Verification items for the finished model (mm, model axes). A direction names the side the tool comes from. Coordinates: 2 decimals unless noted, no trailing zeros. Loops run counter-clockwise (first coordinate to the right, second up) from the corner with the lowest first, then second, coordinate; pieces in that order, holes last. Notation, with made-up numbers: (-15, 16) -> (31, 16) arc R24 cw to (31, 26) -> close; hole circle Ø6 at (75, 9). An arc over 180 degrees is marked (long way). Write item = value, one per line.
```python
from build123d import *

# Parameters (mm, degrees)
CUT_EXTRUDE1_REACH   = 17
CUT_EXTRUDE2_REACH   = 17
CUT_EXTRUDE3_REACH   = 17
CUT_EXTRUDE4_REACH   = 16.83
M8_CLEARANCE_HOLE1_D = 8.917
CHAMFER1_SIZE        = 0.5415
FILLET1_R            = 0.3
FILLET2_R            = 1


with BuildPart() as part:
    # Sketch1 → Revolve1 (revolve)
    with BuildSketch(Plane(origin=(0, 0, 0), x_dir=(-1, 0, 0), z_dir=(0, 0, -1)), mode=Mode.PRIVATE) as revolve1_sk:
        Polygon((-5, 8), (-5, 0), (0, 0), (0, 10), (-3.701184814, 10), align=None)
    revolve(revolve1_sk.sketch.rotate(Axis((5, 0, 0), (-1, 0, 0)), 270), axis=Axis((5, 0, 0), (-1, 0, 0)))

    # Cut-Extrude1: up to this cone (the profile starts inside it)
    cut_extrude1_end = Plane(origin=(0, 0, 0), z_dir=(-1, 0, 0)).offset(-10.195259746) * Cone(1.54e-06, 66.821801925, 43.394584565, align=(Align.CENTER, Align.CENTER, Align.MIN), mode=Mode.PRIVATE)
    # Sketch2 → Cut-Extrude1 (cut, up to the surface)
    with BuildSketch(Plane.ZY, mode=Mode.PRIVATE) as cut_extrude1_sk1:
        with BuildLine():
            Line((9.743587635, 2.25), (8.2, 2.25))
            Line((8.2, 2.25), (8.2, -2.25))
            Line((8.2, -2.25), (9.743587635, -2.25))
            ThreePointArc((9.743587635, -2.25), (10, 0), (9.743587635, 2.25))
        make_face()
    cut_extrude1_tool1 = extrude(cut_extrude1_sk1.sketch, amount=-CUT_EXTRUDE1_REACH, mode=Mode.PRIVATE) & cut_extrude1_end
    add(cut_extrude1_tool1.solids().sort_by_distance((0, 0, 9.059184))[0], mode=Mode.SUBTRACT)

    # Cut-Extrude2: up to this cone (the profile starts inside it)
    cut_extrude2_end = Plane(origin=(0, 0, 0), z_dir=(-1, 0, 0)).offset(-10.195259746) * Cone(1.54e-06, 66.821801925, 43.394584565, align=(Align.CENTER, Align.CENTER, Align.MIN), mode=Mode.PRIVATE)
    # Sketch3 → Cut-Extrude2 (cut, up to the surface)
    with BuildSketch(Plane.ZY, mode=Mode.PRIVATE) as cut_extrude2_sk1:
        with BuildLine():
            Line((2.25, -9.743587635), (2.25, -8.2))
            Line((2.25, -8.2), (-2.25, -8.2))
            Line((-2.25, -8.2), (-2.25, -9.743587635))
            ThreePointArc((-2.25, -9.743587635), (0, -10), (2.25, -9.743587635))
        make_face()
    cut_extrude2_tool1 = extrude(cut_extrude2_sk1.sketch, amount=-CUT_EXTRUDE2_REACH, mode=Mode.PRIVATE) & cut_extrude2_end
    add(cut_extrude2_tool1.solids().sort_by_distance((0, -9.059184, 0))[0], mode=Mode.SUBTRACT)

    # Cut-Extrude3: up to this cone (the profile starts inside it)
    cut_extrude3_end = Plane(origin=(0, 0, 0), z_dir=(-1, 0, 0)).offset(-10.195259746) * Cone(1.54e-06, 66.821801925, 43.394584565, align=(Align.CENTER, Align.CENTER, Align.MIN), mode=Mode.PRIVATE)
    # Sketch4 → Cut-Extrude3 (cut, up to the surface)
    with BuildSketch(Plane.ZY, mode=Mode.PRIVATE) as cut_extrude3_sk1:
        with BuildLine():
            Line((-9.743587635, -2.25), (-8.2, -2.25))
            Line((-8.2, -2.25), (-8.2, 2.25))
            Line((-8.2, 2.25), (-9.743587635, 2.25))
            ThreePointArc((-9.743587635, 2.25), (-10, 0), (-9.743587635, -2.25))
        make_face()
    cut_extrude3_tool1 = extrude(cut_extrude3_sk1.sketch, amount=-CUT_EXTRUDE3_REACH, mode=Mode.PRIVATE) & cut_extrude3_end
    add(cut_extrude3_tool1.solids().sort_by_distance((0, 0, -9.059184))[0], mode=Mode.SUBTRACT)

    # Cut-Extrude4: up to this cone (the profile starts inside it)
    cut_extrude4_end = Plane(origin=(0, 0, 0), z_dir=(-1, 0, 0)).offset(-10.195259746) * Cone(1.54e-06, 66.560024881, 43.224584565, align=(Align.CENTER, Align.CENTER, Align.MIN), mode=Mode.PRIVATE)
    # Sketch5 → Cut-Extrude4 (cut, up to the surface)
    with BuildSketch(Plane.ZY, mode=Mode.PRIVATE) as cut_extrude4_sk1:
        with BuildLine():
            Line((-2.25, 9.743587635), (-2.25, 8.2))
            Line((-2.25, 8.2), (2.25, 8.2))
            Line((2.25, 8.2), (2.25, 9.743587635))
            ThreePointArc((2.25, 9.743587635), (0, 10), (-2.25, 9.743587635))
        make_face()
    cut_extrude4_tool1 = extrude(cut_extrude4_sk1.sketch, amount=-CUT_EXTRUDE4_REACH, mode=Mode.PRIVATE) & cut_extrude4_end
    add(cut_extrude4_tool1.solids().sort_by_distance((0, 9.059184, 0))[0], mode=Mode.SUBTRACT)

    # M8 Clearance Hole1 (through all)
    with Locations(Plane(origin=(5, 0, 0), x_dir=(0, 0, -1), z_dir=(1, 0, 0))):
        with Locations((0, 0)):
            Hole(M8_CLEARANCE_HOLE1_D / 2)

    # Chamfer1
    chamfer1_edges = [part.edges().sort_by_distance(p)[0] for p in [
        (5, 0, -4.4585),
        (0, 0, -4.4585),
    ]]
    chamfer(chamfer1_edges, length=CHAMFER1_SIZE)

    # Fillet1
    fillet1_edges = [part.edges().sort_by_distance(p)[0] for p in [
        (2.336645522, 8.2, -2.25),
        (2.336645522, 2.25, 8.2),
        (2.336645522, -8.2, 2.25),
        (2.336645522, -2.25, 8.2),
        (2.336645522, 8.2, 2.25),
        (2.336645522, -8.2, -2.25),
        (2.336645522, 2.25, -8.2),
        (2.336645522, -2.25, -8.2),
    ]]
    fillet(fillet1_edges, radius=FILLET1_R)

    # Fillet2
    fillet2_edges = [part.edges().sort_by_distance(p)[0] for p in [
        (0, -7.071067812, 7.071067812),
        (0, -7.071067812, -7.071067812),
        (0, 7.071067812, 7.071067812),
        (0, 7.071067812, -7.071067812),
    ]]
    fillet(fillet2_edges, radius=FILLET2_R)


solid = part.part
```
1) Depth check by flat-ended pin: pin 1 Ø3 at (x, z) = (4.5, -5) entering from +Y; pin 2 Ø4 at (y, z) = (-4, -1.5) entering from +X; pin 3 Ø3 at (x, y) = (2, 0) entering from +Z; pin 4 Ø0.6 at (x, y) = (3, 9) entering from -Z. Enter the tip coordinate at first touch or a pass-through.
Ans:
pin_1 = 9.28
pin_2 = 5
pin_3 = 8.2
pin_4 = -4.93
2) Sectioned sample at A-A, the plane y = 0. Record the cut outline in (x, z), plus the area to 3 significant figures.
Ans:
outline = (0, -8.2) -> (4.87, -8.2) -> (5, -8) -> (5, -5) -> (4.46, -4.46) -> (0.54, -4.46) -> (0, -5) -> close; (0, 5) -> (0.54, 4.46) -> (4.46, 4.46) -> (5, 5) -> (5, 8) -> (4.87, 8.2) -> (0, 8.2) -> close
area = 36.8 mm2
3) Material ranges on line 1 (Y direction, x = 2.45, z = 0); line 2 (Y direction, x = 2.5, z = 8.5); line 3 (Z direction, x = 1.8, y = 0.25), recorded low to high.
Ans:
line_1 = -8.2 to -4.46, 4.46 to 8.2
line_2 = -5.27 to -2.25, 2.25 to 5.27
line_3 = -8.2 to -4.45, 4.45 to 8.2
4) Sectioned sample at C-C, the plane x = 4. Record the cut outline in (y, z).
Ans:
outline = (-9.27, -2.25) arc R9.54 ccw to (-2.25, -9.27) -> (-2.25, -8.5) arc R0.3 cw to (-1.95, -8.2) -> (1.95, -8.2) arc R0.3 cw to (2.25, -8.5) -> (2.25, -9.27) arc R9.54 ccw to (9.27, -2.25) -> (8.5, -2.25) arc R0.3 cw to (8.2, -1.95) -> (8.2, 1.95) arc R0.3 cw to (8.5, 2.25) -> (9.27, 2.25) arc R9.54 ccw to (2.25, 9.27) -> (2.25, 8.5) arc R0.3 cw to (1.95, 8.2) -> (-1.95, 8.2) arc R0.3 cw to (-2.25, 8.5) -> (-2.25, 9.27) arc R9.54 ccw to (-9.27, 2.25) -> (-8.5, 2.25) arc R0.3 cw to (-8.2, 1.95) -> (-8.2, -1.95) arc R0.3 cw to (-8.5, -2.25) -> close; hole circle Ø8.92 at (0, 0)
5) Tool access check on faces 4 (the face through (2, -8.2, 0)), 5 (the face through (2, 9, -2.25)), 6 (the face through (2, 0, -8.2)), 7 (the face through (2, 2.25, 9)). Record the directions out of +Z, -Z, +X, -X, +Y, -Y that give a thin tool (end or side, any length) a straight path to the whole face; none if there is none.
Ans:
face_4 = +X, -X, -Y
face_5 = +X, -X, +Y
face_6 = -Z, +X, -X
face_7 = +Z, +X, -X
6) Release check for a two-part mould opening along Y. For faces 1 (the face through (2, -9, -2.25)), 2 (the face through (2.47, -2.71, -3.54)), 3 (the face through (2.37, 7.016, 7.126)) record: pulls with the +Y half, pulls with the -Y half, needs draft (parallel to the pull), parting line crosses it, or undercut.
Ans:
face_1 = needs draft
face_2 = undercut
face_3 = pulls with the +Y half
7) Sectioned sample at D-D, the plane x = 1.85. Record the cut outline in (y, z), plus the area to 3 significant figures.
Ans:
outline = (-9.74, -2.25) arc R10 ccw to (-2.25, -9.74) -> (-2.25, -8.5) arc R0.3 cw to (-1.95, -8.2) -> (1.95, -8.2) arc R0.3 cw to (2.25, -8.5) -> (2.25, -9.74) arc R10 ccw to (9.74, -2.25) -> (8.5, -2.25) arc R0.3 cw to (8.2, -1.95) -> (8.2, 1.95) arc R0.3 cw to (8.5, 2.25) -> (9.74, 2.25) arc R10 ccw to (2.25, 9.74) -> (2.25, 8.5) arc R0.3 cw to (1.95, 8.2) -> (-1.95, 8.2) arc R0.3 cw to (-2.25, 8.5) -> (-2.25, 9.74) arc R10 ccw to (-9.74, 2.25) -> (-8.5, 2.25) arc R0.3 cw to (-8.2, 1.95) -> (-8.2, -1.95) arc R0.3 cw to (-8.5, -2.25) -> close; hole circle Ø8.92 at (0, 0)
area = 221 mm2
